```python
from build123d import *

# Parameters (mm, degrees)
SKETCH2_W           = 42.3
SKETCH2_H           = 42.3
SKETCH2_R           = 1.5
SKETCH2_R_2         = 12
BOSS_EXTRUDE1_DEPTH = 5
SKETCH3_W           = 55
SKETCH3_H           = 100
SKETCH3_R           = 2.75
SKETCH3_W_2         = 15
SKETCH3_H_2         = 17.5
BOSS_EXTRUDE2_DEPTH = 5
FILLET1_R           = 5


with BuildPart() as part:
    # Sketch2 → Boss-Extrude1 (new body)
    with BuildSketch(Plane(origin=(0, 0, 0), x_dir=(0, 0, -1), z_dir=(1, 0, 0))):
        Rectangle(SKETCH2_W, SKETCH2_H)
        with Locations((-15.5, 15.5)):
            Circle(SKETCH2_R, mode=Mode.SUBTRACT)
        with Locations((15.5, 15.5)):
            Circle(SKETCH2_R, mode=Mode.SUBTRACT)
        with Locations((15.5, -15.5)):
            Circle(SKETCH2_R, mode=Mode.SUBTRACT)
        with Locations((-15.5, -15.5)):
            Circle(SKETCH2_R, mode=Mode.SUBTRACT)
        Circle(SKETCH2_R_2, mode=Mode.SUBTRACT)
    extrude(amount=BOSS_EXTRUDE1_DEPTH)

    # Sketch3 → Boss-Extrude2 (add)
    with BuildSketch(Plane.XY.offset(21.15)):
        with Locations((27.5, 20)):
            Rectangle(SKETCH3_W, SKETCH3_H)
        with Locations((50, -25)):
            Circle(SKETCH3_R, mode=Mode.SUBTRACT)
        with Locations((10, -25)):
            Circle(SKETCH3_R, mode=Mode.SUBTRACT)
        with Locations((20, 11.25)):
            Rectangle(SKETCH3_W_2, SKETCH3_H_2, mode=Mode.SUBTRACT)
        with Locations((40, 11.25)):
            Rectangle(SKETCH3_W_2, SKETCH3_H_2, mode=Mode.SUBTRACT)
        with Locations((40, -11.25)):
            Rectangle(SKETCH3_W_2, SKETCH3_H_2, mode=Mode.SUBTRACT)
        with Locations((20, -11.25)):
            Rectangle(SKETCH3_W_2, SKETCH3_H_2, mode=Mode.SUBTRACT)
        with BuildLine():
            Line((50.75, 63), (50.75, 38))
            ThreePointArc((50.75, 38), (48, 35.25), (45.25, 38))
            Line((45.25, 38), (45.25, 63))
            ThreePointArc((45.25, 63), (48, 65.75), (50.75, 63))
        make_face(mode=Mode.SUBTRACT)
        with BuildLine():
            Line((12.75, 63), (12.75, 38))
            ThreePointArc((12.75, 38), (10, 35.25), (7.25, 38))
            Line((7.25, 38), (7.25, 63))
            ThreePointArc((7.25, 63), (10, 65.75), (12.75, 63))
        make_face(mode=Mode.SUBTRACT)
    extrude(amount=BOSS_EXTRUDE2_DEPTH)

    # Fillet1
    fillet1_edges = [part.edges().sort_by_distance(p)[0] for p in [
        (2.5, -21.15, 21.15),
        (2.5, 21.15, 21.15),
    ]]
    fillet(fillet1_edges, radius=FILLET1_R)


solid = part.part
```
Can you work these out from the model? Positions are in its coordinate system, mm. A direction names the side the tool comes from. Round coordinates to 2 decimals unless told otherwise and drop trailing zeros. Order: outer loops, then holes, each group sorted by start corner. A loop starts at its lowest first (then second) coordinate and runs counter-clockwise, first axis right, second up. Notation, with made-up numbers: (-16, 25) -> (30, 25) arc R22 ccw to (30, 56) -> close; hole circle Ø7 at (68, 77). An arc over 180 degrees is marked (long way). Return JSON: item names as keys, results as strings. Group by question number.
1. We'd pull the mould along Y, two halves only. Please class faces 1 (the face through (7.25, 50, 24)), 2 (the face through (2.54, -22.65, 19.72)), 3 (the face through (27, 70, 24)), 4 (the face through (47.5, -11, 24)): released by +Y, released by -Y, zero draft, split by the parting line, or undercut.
2. If we section it at B-B, the plane z = 22.5: Count the separate pieces of the cut face and the enclosed holes in it, then the cut area to 3 significant figures.
3. Which directions (+Z, -Z, +X, -X, +Y, -Y) give clear straight access to the entire face, cutting with the end or side of a thin tool? Please do faces 5 (the face through (27.5, 11, 24)), 6 (the face through (0, 8, 13)).
4. If we section it at C-C, the plane y = 15.5: Write out the boundary of the cut face in (x, z).
5. If we section it at D-D, the plane z = -15.5: Write out the boundary of the cut face in (x, y), then the cut area to 4 significant figures.
6. I need wall thicknesses on line 1 (Y direction, x = 2.05, z = -15.5); line 2 (X direction, y = 13.5, z = 22); line 3 (Z direction, x = 1, y = 15). Which ranges of each line are inside material? Lowest first, please. Write a range as [from, to].
7. Will these pins go through, and if not, where does the flat tip stop? pin 1 (16.5 mm diameter, centred on x = 32, y = 37, fed in from -Z); pin 2 (5 mm diameter, centred on y = -15.5, z = -15.5, fed in from +X); pin 3 (5.5 mm diameter, centred on x = 2, z = -6, fed in from -Y).
8. If we section it at A-A, the plane x = 10: Write out the boundary of the cut face in (y, z), then the cut area to 3 significant figures.
Output values:
{
 "1": {"face 1": "undercut", "face 2": "released by -Y", "face 3": "released by +Y", "face 4": "undercut"},
 "2": {"separate pieces": "1", "enclosed holes": "8", "area": "4,080 mm²"},
 "3": {"face 5": "+Z, -Z", "face 6": "+Z, -Z, -X, +Y, -Y"},
 "4": {"outline": "(0, -21.15) -> (5, -21.15) -> (5, -17) -> (0, -17) -> close; (0, -14) -> (5, -14) -> (5, 14) -> (0, 14) -> close; (0, 17) -> (5, 17) -> (5, 21.15) -> (12.5, 21.15) -> (12.5, 26.15) -> (0, 26.15) -> close; (27.5, 21.15) -> (32.5, 21.15) -> (32.5, 26.15) -> (27.5, 26.15) -> close; (47.5, 21.15) -> (55, 21.15) -> (55, 26.15) -> (47.5, 26.15) -> close"},
 "5": {"outline": "(0, -21.15) -> (5, -21.15) -> (5, -17) -> (0, -17) -> close; (0, -14) -> (5, -14) -> (5, 14) -> (0, 14) -> close; (0, 17) -> (5, 17) -> (5, 21.15) -> (0, 21.15) -> close", "area": "181.5 mm²"},
 "6": {"line 1": "[-21.15, -17], [-14, 14], [17, 21.15]", "line 2": "[0, 12.5], [27.5, 32.5], [47.5, 55]", "line 3": "[-21.15, -16.91], [-14.09, 14.09], [16.91, 26.15]"},
 "7": {"pin 1": "z = 21.15", "pin 2": "x = 5", "pin 3": "y = -21.15"},
 "8": {"outline": "(-30, 21.15) -> (-27.75, 21.15) -> (-27.75, 26.15) -> (-30, 26.15) -> close; (-22.25, 21.15) -> (35.25, 21.15) -> (35.25, 26.15) -> (-22.25, 26.15) -> close; (65.75, 21.15) -> (70, 21.15) -> (70, 26.15) -> (65.75, 26.15) -> close", "area": "320 mm²"}
}
